from build123d import *

# Parameters (mm, degrees)
SKETCH1_W           = 195.072
SKETCH1_H           = 152.4
BOSS_EXTRUDE1_DEPTH = 2.54
SKETCH2_R           = 1.5875
SKETCH2_R_2         = 1.5
SKETCH2_R_3         = 2.54
SKETCH2_W           = 36.254936194
SKETCH2_H           = 46.345137013
CUT_EXTRUDE1_DEPTH  = 2.54
CUT_EXTRUDE2_DEPTH  = 2.54
SKETCH6_R           = 1.5875
BOSS_EXTRUDE2_DEPTH = 15.24


with BuildPart() as part:
    # Sketch1 → Boss-Extrude1 (new body)
    with BuildSketch(Plane(origin=(0, 0, 0), x_dir=(1, 0, 0), z_dir=(0, 1, 0))):
        with Locations((97.536, 76.2)):
            Rectangle(SKETCH1_W, SKETCH1_H)
    extrude(amount=BOSS_EXTRUDE1_DEPTH)

    # Sketch2 → Cut-Extrude1 (cut)
    with BuildSketch(Plane(origin=(0, 2.54, 0), x_dir=(1, 0, 0), z_dir=(0, 1, 0))):
        with Locations((56.571242474, 139.7)):
            Circle(SKETCH2_R)
        with Locations((139.121242474, 139.7)):
            Circle(SKETCH2_R)
        with Locations((139.121242474, 81.28)):
            Circle(SKETCH2_R)
        with Locations((56.571242474, 81.28)):
            Circle(SKETCH2_R)
        with Locations((186, 61.35)):
            Circle(SKETCH2_R_2)
        with Locations((186, 86.35)):
            Circle(SKETCH2_R_2)
        with Locations((186, 111.35)):
            Circle(SKETCH2_R_2)
        with Locations((9, 111.35)):
            Circle(SKETCH2_R_2)
        with Locations((9, 86.35)):
            Circle(SKETCH2_R_2)
        with Locations((9, 61.35)):
            Circle(SKETCH2_R_2)
        with Locations((56.571242474, 46.705739829)):
            Circle(SKETCH2_R_3)
        with Locations((33.737644143, 61.35)):
            Circle(SKETCH2_R_3)
        with Locations((161.334355857, 61.35)):
            Circle(SKETCH2_R_3)
        with Locations((138.500757526, 46.705739829)):
            Circle(SKETCH2_R_3)
        with Locations((97.536, 12.019328057)):
            Rectangle(SKETCH2_W, SKETCH2_H)
    extrude(amount=-CUT_EXTRUDE1_DEPTH, mode=Mode.SUBTRACT)

    # Sketch4 → Cut-Extrude2 (cut)
    with BuildSketch(Plane(origin=(0, 2.54, 0), x_dir=(1, 0, 0), z_dir=(0, 1, 0))):
        with BuildLine():
            Line((195.072, 51.488555228), (195, 51.488555228))
            ThreePointArc((195, 51.488555228), (157.216035085, 31.583435817), (115.663468097, 21.723113302))
            Line((115.663468097, 21.723113302), (115.663468097, 0))
            Line((115.663468097, 0), (195.072, 0))
            Line((195.072, 0), (195.072, 51.488555228))
        make_face()
        with BuildLine():
            ThreePointArc((79.408531903, 21.715391762), (37.817865405, 31.570721166), (0, 51.488555228))
            Line((0, 51.488555228), (0, 0))
            Line((0, 0), (79.408531903, 0))
            Line((79.408531903, 0), (79.408531903, 21.715391762))
        make_face()
    extrude(amount=-CUT_EXTRUDE2_DEPTH, mode=Mode.SUBTRACT)

    # Sketch6 → Boss-Extrude2 (add)
    with BuildSketch(Plane(origin=(0, 2.54, 0), x_dir=(1, 0, 0), z_dir=(0, 1, 0))):
        with BuildLine():
            Line((60.970651525, 142.24), (52.171833423, 142.24))
            ThreePointArc((52.171833423, 142.24), (55.256441725, 134.793096802), (61.651242474, 139.7))
            ThreePointArc((61.651242474, 139.7), (61.478145672, 141.014800749), (60.970651525, 142.24))
        make_face()
        with Locations((56.571242474, 139.7)):
            Circle(SKETCH6_R, mode=Mode.SUBTRACT)
        with BuildLine():
            ThreePointArc((144.201242474, 139.7), (144.028145672, 141.014800749), (143.520651525, 142.24))
            Line((143.520651525, 142.24), (134.721833423, 142.24))
            ThreePointArc((134.721833423, 142.24), (137.806441725, 134.793096802), (144.201242474, 139.7))
        make_face()
        with Locations((139.121242474, 139.7)):
            Circle(SKETCH6_R, mode=Mode.SUBTRACT)
        with BuildLine():
            Line((134.721833423, 78.74), (143.520651525, 78.74))
            ThreePointArc((143.520651525, 78.74), (144.028145672, 79.965199251), (144.201242474, 81.28))
            ThreePointArc((144.201242474, 81.28), (137.806441725, 86.186903198), (134.721833423, 78.74))
        make_face()
        with Locations((139.121242474, 81.28)):
            Circle(SKETCH6_R, mode=Mode.SUBTRACT)
        with BuildLine():
            ThreePointArc((61.651242474, 81.28), (55.256441725, 86.186903198), (52.171833423, 78.74))
            Line((52.171833423, 78.74), (60.970651525, 78.74))
            ThreePointArc((60.970651525, 78.74), (61.478145672, 79.965199251), (61.651242474, 81.28))
        make_face()
        with Locations((56.571242474, 81.28)):
            Circle(SKETCH6_R, mode=Mode.SUBTRACT)
    extrude(amount=BOSS_EXTRUDE2_DEPTH)


solid = part.part
Design review of the part built by this model. Coordinates are the model's own, in mm. A direction names the side the tool comes from. Coordinates: 2 decimals unless noted, no trailing zeros. Order: outer loops, then holes, each group sorted by start corner. A loop starts at its lowest first (then second) coordinate and runs counter-clockwise, first axis right, second up. Notation, with made-up numbers: (66.5, -36.75) -> (74.5, -36.75) arc R19 ccw to (74.5, -23.75) -> close; hole circle Ø1 at (85, -9). An arc over 180 degrees is marked (long way). Use one line per item in the form item = value. Start each with the question number.
(1) Add section C-C on x = 102. State the section outline as (y, z) points.
(2) For faces 1 (the flat face through (140, 17.78, -138)), 2 (the flat face through (139, 10, -142.24)), 3 (the flat face through (57, 10, -78.74)), list the 3-axis set-ups (+Z, -Z, +X, -X, +Y, -Y) from which the entire face can be reached by the end or side of a thin tool; tool diameter is ignored.
(3) Insertion check: pin 1 (2.5 mm diameter, centred on x = 56, y = 9, fed in from -Z); pin 2 (7 mm diameter, centred on x = 55, y = 12, fed in from +Z); pin 3 (1 mm diameter, centred on x = 121.5, z = -136.5, fed in from +Y). Each pin has a flat end and moves straight along its axis. Give the tip position at first contact, or say it passes through.
(4) Add section D-D on z = -67. State the section outline as (x, y) points.
(5) Add section A-A on y = 13.25. State the section outline as (x, z) points (1 decimal).
(6) Add section B-B on z = -32.5. State the section outline as (x, y) points.
(7) For probe 1 along X at (y, z) = (1.35, -81.28); probe 2 along X at (y, z) = (0.55, -61.35); probe 3 along X at (y, z) = (9.5, -81.28), list the stretches that pass through material, from the lowest coordinate up.
Answer block:
q1.outline = (0, -152.4) -> (2.54, -152.4) -> (2.54, -35.19) -> (0, -35.19) -> close
q2.face_1 = +Z, -Z, +X, -X, +Y
q2.face_2 = -Z, +X, -X, +Y
q2.face_3 = +Z, +X, -X, +Y
q3.pin_1 = -142.24
q3.pin_2 = -78.74
q3.pin_3 = 2.54
q4.outline = (0, 0) -> (195.07, 0) -> (195.07, 2.54) -> (0, 2.54) -> close
q5.outline = (52.2, -142.2) -> (61, -142.2) arc R5.1 ccw (long way) to start; (52.2, -78.7) arc R5.1 ccw (long way) to (61, -78.7) -> close; (134.7, -142.2) -> (143.5, -142.2) arc R5.1 ccw (long way) to start; (134.7, -78.7) arc R5.1 ccw (long way) to (143.5, -78.7) -> close; hole circle Ø3.2 at (56.6, -139.7); hole circle Ø3.2 at (56.6, -81.3); hole circle Ø3.2 at (139.1, -139.7); hole circle Ø3.2 at (139.1, -81.3)
q6.outline = (35.4, 0) -> (79.41, 0) -> (79.41, 2.54) -> (35.4, 2.54) -> close; (115.66, 0) -> (159.6, 0) -> (159.6, 2.54) -> (115.66, 2.54) -> close
q7.probe_1 = 0 to 54.98, 58.16 to 137.53, 140.71 to 195.07
q7.probe_2 = 0 to 7.5, 10.5 to 31.2, 36.28 to 158.79, 163.87 to 184.5, 187.5 to 195.07
q7.probe_3 = 51.49 to 54.98, 58.16 to 61.65, 134.04 to 137.53, 140.71 to 144.2
